Part model, mm, in its own coordinate system. A direction names the side the tool comes from. Coordinates: 2 decimals unless noted, no trailing zeros. Loops run counter-clockwise (first coordinate to the right, second up) from the corner with the lowest first, then second, coordinate; pieces in that order, holes last. Notation, with made-up numbers: (31.5, 82.5) -> (40.5, 82.5) arc R13 ccw to (40.5, 86.5) -> close; hole circle Ø11 at (86, 85.5). An arc over 180 degrees is marked (long way). Use one line per item in the form item = value. Start each with the question number.
(1) Mould opens along Z. For faces 5 (the cylindrical face through (-0.239, 4.86, 18.504)), 6 (the flat face through (0, 5, -5.6)), 7 (the flat face through (0, 15, -4)) say: +Z half, -Z half, draft (parallel to the pull), parting line (faces both ways), or undercut.
(2) 3-axis set-ups, long thin cutter, end or side, ignore diameter. For faces 1 (the flat face through (0, 5, 30.672)), 2 (the flat face through (-2.5, 5, 11)), 3 (the flat face through (5.289, 0.688, 0.036)), 4 (the cylindrical face through (0.29, -2.73, 32.07)): which of +Z, -Z, +X, -X, +Y, -Y reach the whole face in a straight line?
(3) Band-saw the part on B-B on z = 25. Give the cut face in (x, y).
(4) Pin check, flat tips, straight feed: P1, Ø12, axis at y = -0.5, z = 14, coming from the -X side; P2, Ø8, axis at x = 5, y = 1.5, coming from the +Z side; P3, Ø1, axis at x = 0, z = 20.5, coming from the +Y side; P4, Ø2.5, axis at x = 0, z = 13.5, coming from the -Y side. Stop position of each tip, or through.
(5) Band-saw the part on A-A on y = 5.75. Give the cut face in (x, z) (3 decimals).
(6) Band-saw the part on C-C on x = -5.25. Give the cut face in (y, z), then the cut area to 3 significant figures.
(7) Drill centre lines: L1, parallel to Y at x = 0, z = 31.8; L2, parallel to Z at x = 0, y = 13.75; L3, parallel to Z at x = 9, y = 9.25. Where is each one in solid material? Low to high. Write a range as [from, to].
(8) Band-saw the part on D-D on x = -8. Give the cut face in (y, z).
```python
from build123d import *

# Parameters (mm, degrees)
SKETCH2_W                       = 20
SKETCH2_H                       = 10
BOSS_EXTRUDE1_DEPTH             = 2.6
CHAMFER1_SIZE                   = 9.5
CHAMFER1_SIZE2                  = 8.553838421
FILLET3_R                       = 1
SKETCH3_W                       = 20
SKETCH3_H                       = 20
BOSS_EXTRUDE2_DEPTH             = 3
BOSS_EXTRUDE3_REACH             = 20.877
SKETCH6_R                       = 8.5
BOSS_EXTRUDE3_DIRECTION_2_REACH = 20.877
BOSS_EXTRUDE4_REACH             = 35.218
BOSS_EXTRUDE4_END_RADIUS        = 8.5
SKETCH5_W                       = 5
SKETCH5_H                       = 16
CUT_EXTRUDE1_REACH              = 33.311
CUT_EXTRUDE1_END_RADIUS         = 8.5
SKETCH7_R                       = 2.25


with BuildPart() as part:
    # Sketch2 → Boss-Extrude1 (new, symmetric)
    with BuildSketch(Plane.XY):
        Rectangle(SKETCH2_W, SKETCH2_H)
    extrude(amount=BOSS_EXTRUDE1_DEPTH, both=True)

    # Chamfer1
    chamfer1_edges = [part.edges().sort_by_distance(p)[0] for p in [
        (-10, 5, 0),
        (10, 5, 0),
    ]]
    chamfer1_side = [part.faces().sort_by_distance(p)[0] for p in [
        (0, 5, 0),
    ]]
    chamfer(chamfer1_edges, length=CHAMFER1_SIZE, length2=CHAMFER1_SIZE2, reference=chamfer1_side[0])

    # Fillet3
    fillet3_edges = [part.edges().sort_by_distance(p)[0] for p in [
        (-0.5, 5, 0),
        (0.5, 5, 0),
        (10, -3.553838421, 0),
        (-10, -3.553838421, 0),
    ]]
    fillet(fillet3_edges, radius=FILLET3_R)

    # Sketch3 → Boss-Extrude2 (add)
    with BuildSketch(Plane.XY.offset(2.6)):
        with Locations((0, 5)):
            Rectangle(SKETCH3_W, SKETCH3_H)
    boss_extrude2 = extrude(amount=BOSS_EXTRUDE2_DEPTH)

    # Mirror1: Boss-Extrude2 across plane
    add(boss_extrude2.mirror(Plane.XY))


with BuildPart() as body_2:

    # Boss-Extrude3: up to this face of the body (flat: up to its plane)
    boss_extrude3_end = Plane(part.part.faces().sort_by_distance((0, 15, 4.1))[0])
    # Sketch6 → Boss-Extrude3 (new, up to the picked face)
    with BuildSketch(Plane(origin=(0, 0, 0), x_dir=(1, 0, 0), z_dir=(0, 1, 0)), mode=Mode.PRIVATE) as boss_extrude3_sk1:
        with Locations(Location((0, -25, 0), (0, 0, 90))):
            Circle(SKETCH6_R)
        with BuildLine():
            Line((3.175, -30.671805268), (-3.175, -30.671805268))
            ThreePointArc((-3.175, -30.671805268), (0, -18.5), (3.175, -30.671805268))
        make_face(mode=Mode.SUBTRACT)
    boss_extrude3_tool1 = split(extrude(boss_extrude3_sk1.sketch, amount=BOSS_EXTRUDE3_REACH, mode=Mode.PRIVATE), bisect_by=boss_extrude3_end, keep=Keep.BOTH, mode=Mode.PRIVATE)
    add(boss_extrude3_tool1.solids().sort_by(Axis((0, 0, 33.259584), (0, 1, 0)))[0])


    # Boss-Extrude3 direction 2: up to this face of the body (flat: up to its plane)
    boss_extrude3_direction_2_end = Plane(part.part.faces().sort_by_distance((0, -5, 0))[0])
    # Sketch6 → Boss-Extrude3 direction 2 (add, up to the picked face)
    with BuildSketch(Plane(origin=(0, 0, 0), x_dir=(1, 0, 0), z_dir=(0, 1, 0)), mode=Mode.PRIVATE) as boss_extrude3_direction_2_sk1:
        with Locations(Location((0, -25, 0), (0, 0, 90))):
            Circle(SKETCH6_R)
        with BuildLine():
            Line((3.175, -30.671805268), (-3.175, -30.671805268))
            ThreePointArc((-3.175, -30.671805268), (0, -18.5), (3.175, -30.671805268))
        make_face(mode=Mode.SUBTRACT)
    boss_extrude3_direction_2_tool1 = split(extrude(boss_extrude3_direction_2_sk1.sketch, amount=-BOSS_EXTRUDE3_DIRECTION_2_REACH, mode=Mode.PRIVATE), bisect_by=boss_extrude3_direction_2_end, keep=Keep.BOTH, mode=Mode.PRIVATE)
    add(boss_extrude3_direction_2_tool1.solids().sort_by(Axis((0, 0, 33.259584), (0, -1, 0)))[0])


with BuildPart() as part_1:
    add(part.part)

    add(body_2.part)  # Boss-Extrude4 merges body 2
    # Boss-Extrude4: up to this cylinder (the profile starts outside it)
    boss_extrude4_end = Plane(origin=(0, 5, 25), z_dir=(0, -1, 0)) * Cylinder(BOSS_EXTRUDE4_END_RADIUS, 88.436, mode=Mode.PRIVATE)
    # Sketch5 → Boss-Extrude4 (add, up to the surface)
    with BuildSketch(Plane.XY.offset(5.6), mode=Mode.PRIVATE) as boss_extrude4_sk1:
        with Locations((0, 5)):
            Rectangle(SKETCH5_W, SKETCH5_H)
    boss_extrude4_tool1 = extrude(boss_extrude4_sk1.sketch, amount=BOSS_EXTRUDE4_REACH, mode=Mode.PRIVATE) - boss_extrude4_end
    add(boss_extrude4_tool1.solids().sort_by_distance((0, 5, 5.6))[0])

    # Cut-Extrude1: up to this cylinder (the profile starts inside it)
    cut_extrude1_end = Plane(origin=(0, 5, 25), z_dir=(0, -1, 0)) * Cylinder(CUT_EXTRUDE1_END_RADIUS, 95.622, mode=Mode.PRIVATE)
    # Sketch7 → Cut-Extrude1 (cut, up to the surface)
    with BuildSketch(Plane.XY.offset(20), mode=Mode.PRIVATE) as cut_extrude1_sk1:
        with Locations(Location((0, 10.5, 0), (0, 0, 180))):
            Circle(SKETCH7_R)
    cut_extrude1_tool1 = extrude(cut_extrude1_sk1.sketch, amount=CUT_EXTRUDE1_REACH, mode=Mode.PRIVATE) & cut_extrude1_end
    add(cut_extrude1_tool1.solids().sort_by_distance((0, 10.5, 20))[0], mode=Mode.SUBTRACT)
    # Sketch7 → Cut-Extrude1 (cut, up to the surface)
    with BuildSketch(Plane.XY.offset(20), mode=Mode.PRIVATE) as cut_extrude1_sk2:
        with Locations(Location((0, -0.5, 0), (0, 0, 180))):
            Circle(SKETCH7_R)
    cut_extrude1_tool2 = extrude(cut_extrude1_sk2.sketch, amount=CUT_EXTRUDE1_REACH, mode=Mode.PRIVATE) & cut_extrude1_end
    add(cut_extrude1_tool2.solids().sort_by_distance((0, -0.5, 20))[0], mode=Mode.SUBTRACT)


solid = part_1.part
```
A:
q1.face_5 = undercut
q1.face_6 = -Z half
q1.face_7 = draft
q2.face_1 = +Y, -Y
q2.face_2 = -X, +Y, -Y
q2.face_3 = +X, +Y
q2.face_4 = +Z
q3.outline = (-8.5, -5) -> (-6.5, -5) -> (-6.5, 15) -> (-8.5, 15) -> close; (6.5, -5) -> (8.5, -5) -> (8.5, 15) -> (6.5, 15) -> close
q4.P1 = -6.87
q4.P2 = 33.44
q4.P3 = through
q4.P4 = -3
q5.outline = (-10, -5.6) -> (10, -5.6) -> (10, -2.6) -> (-10, -2.6) -> close; (-10, 2.6) -> (10, 2.6) -> (10, 5.6) -> (2.5, 5.6) -> (2.5, 16.876) arc R8.5 ccw (long way) to (-2.5, 16.876) -> (-2.5, 5.6) -> (-10, 5.6) -> close; hole (-3.175, 30.672) arc R6.5 ccw (long way) to (3.175, 30.672) -> close
q6.outline = (-5, -5.6) -> (15, -5.6) -> (15, -2.6) -> (0.72, -2.6) -> (0.72, 2.6) -> (15, 2.6) -> (15, 5.6) -> (-5, 5.6) -> close; (-5, 18.32) -> (15, 18.32) -> (15, 21.17) -> (-5, 21.17) -> close; (-5, 28.83) -> (15, 28.83) -> (15, 31.68) -> (-5, 31.68) -> close
q6.area = 264 mm²
q7.L1 = [-5, -2.75], [1.75, 8.25], [12.75, 15]
q7.L2 = [-5.6, -2.6], [2.6, 5.6], [16.5, 18.5], [30.67, 33.5]
q7.L3 = [-5.6, -2.6], [2.6, 5.6]
q8.outline = (-5, -5.6) -> (15, -5.6) -> (15, -2.6) -> (-1.75, -2.6) -> (-1.75, 2.6) -> (15, 2.6) -> (15, 5.6) -> (-5, 5.6) -> close; (-5, 22.13) -> (15, 22.13) -> (15, 27.87) -> (-5, 27.87) -> close
